Autodesk Inventor part; units mm, degrees
ref_plane "YZ Plane" through (0, 0, 0) normal (1, 0, 0) x (0, 1, 0)
ref_plane "XZ Plane" through (0, 0, 0) normal (0, 1, 0) x (-1, 0, 0)
ref_plane "XY Plane" through (0, 0, 0) normal (0, 0, 1) x (1, 0, 0)
sketch "Sketch1" plane through (0, 0, 0) normal (0, 0, 1) x (1, 0, 0)
  line L0 (-20, 10) -> (20, 10)
  line L1 (20, 10) -> (20, -10)
  line L2 (20, -10) -> (-20, -10)
  line L3 (-20, -10) -> (-20, 10)
  line L4 (-20, 10) -> (20, -10) construction
  line L5 (20, 10) -> (-20, -10) construction
  line L6 (18, 8) -> (-18, 8)
  line L7 (-18, 8) -> (-18, -8)
  line L8 (-18, -8) -> (18, -8)
  line L9 (18, -8) -> (18, 8)
  point P0 (0, 0)
  dimension "d0" = 40
  dimension "d1" = 20
  dimension "d2" = 2
extrude "Extrusion1" add sketch "Sketch1" along normal mid plane 1900
sketch "Sketch2" plane through (0, 0, 0) normal (0, 1, 0) x (-1, 0, 0)
  line L0 (20, -950) -> (20, 950)
  line L1 (-20, 950) -> (20, 950)
  line L2 (-20, -950) -> (-20, 950)
  line L3 (20, -950) -> (-20, -950)
  line L4 (-20, -950) -> (-50.7107, -950)
  line L5 (-50.7107, -950) -> (-50.7107, 950)
  line L6 (-50.7107, 950) -> (-20, 950)
  line L7 (20, -879.2893) -> (-50.7107, -950)
  line L8 (20, -879.2893) -> (-20, -862.7208)
  line L9 (-20, -950) -> (-20, 950)
  point P0 (0, 0)
  point P1 (-20, -919.2893)
  dimension "d5" = 45
  dimension "d6" = 100
  dimension "d19" = 67.5
extrude "Extrusion2" cut sketch "Sketch2" along normal through all both and the other way through all contours L3 L2 L7 L0 | L7 L2 L8
mirror "Mirror1" about plane through (0, 0, 0) normal (0, 0, 1) of "Extrusion2"
sketch "Sketch3" plane through (0, 0, 0) normal (0, 1, 0) x (-1, 0, 0)
  line L0 (0, 0) -> (0, -871.0051) construction
  line L1 (-20, -862.7208) -> (-20, 862.7208) construction
  line L2 (-20, -475) -> (20, -475) construction
  line L3 (20, 879.2893) -> (20, -879.2893) construction
  circle A0 centre (0, -100) radius 5.5
  circle A1 centre (0, -375) radius 5.5
  circle A2 centre (0, -575) radius 5.5
  circle A3 centre (0, -850) radius 5.5
  line L4 (20, 879.2893) -> (20, -879.2893) construction
  line L5 (-20, -862.7208) -> (20, -879.2893) construction
  dimension "d9" = 475
  dimension "d10" = 11
  dimension "d11" = 275
  dimension "d12" = 275
  dimension "d13" = 100
  dimension "d14" = 100
  dimension "d15" = 100
extrude "Extrusion3" cut sketch "Sketch3" along normal through all
sketch "Sketch5" plane through (-20, -10, -879.2893) normal (0, -1, 0) x (1, 0, 0)
  line L0 (40, 1742.0101) -> (0, 1758.5786) construction
  line L1 (0, 1758.5786) -> (0, 0) construction
  line L2 (0, 0) -> (40, 16.5685) construction
  line L3 (40, 16.5685) -> (40, 1742.0101) construction
  circle A0 centre (20, 114.2893) radius 5.5
  circle A1 centre (20, 760.7893) radius 5.5
  circle A2 centre (20, 285.7893) radius 5.5
  circle A3 centre (20, 522.7893) radius 5.5
  line L4 (20, 522.7893) -> (20, 285.7893) construction
  point P0 (20, 879.2893)
  point P1 (20, 8.2843)
  point P2 (20, 404.2893)
  dimension "d20" = 765
  dimension "d21" = 11
  dimension "d24" = 11
  dimension "d25" = 118.5
  dimension "d26" = 237
  dimension "d27" = 475
extrude "Extrusion4" cut sketch "Sketch5" against normal up to surface (2 mm away)
mirror "Mirror2" about plane through (0, 0, 0) normal (0, 0, 1) of "Extrusion3", "Extrusion4"
fillet "Fillet1" radius 2 4 edges at (-20, 10, 0) (-20, -10, 0) (20, -10, 0) (20, 10, 0)
equation "\"d19\" = 1.5 * d5"
equation "\"d11\" = d12"
equation "\"d13\" = d15"
equation "\"d14\" = d15"
properties part number "Long tube 1"
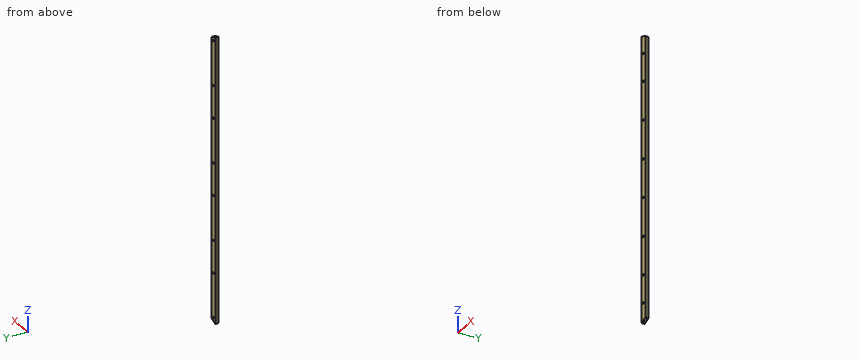
Verification items for the finished model (mm, model axes). Round coordinates to 2 decimals unless told otherwise and drop trailing zeros. Order: outer loops, then holes, each group sorted by start corner. A loop starts at its lowest first (then second) coordinate and runs counter-clockwise, first axis right, second up. Notation, with made-up numbers: (25.5, -21) - (83.5, -21) arc R33 ccw to (83.5, 9) - close; hole circle Ø9 at (21, -25.5). An arc over 180 degrees is marked (long way). Use CSV: the item, a comma, the result in double quotes. Start each with the question number.
1) Go/stop test with flat-tipped pins: P1, Ø10, axis at x = 0, z = -118.5, coming from the -Y side; P2, Ø9, axis at x = 0, z = 100, coming from the +Y side. Record where each tip stops, or that it passes through.
2) Thickness scan on L1, parallel to X at y = -7.75, z = -23; L2, parallel to Y at x = 17, z = 270.5; L3, parallel to X at y = 8.7, z = -850. Record the ranges inside material, lowest first.
3) Section check B-B, the plane z = -688.5. Record the cut outline in (x, y), plus the area to 3 significant figures.
4) Section check A-A, the plane y = -3.5. Record the cut outline in (x, z), plus the area to 3 significant figures.
Answers:
1,P1,"stops at y = 8"
1,P2,"stops at y = -8"
2,L1,"x = -20 to -18, 18 to 20"
2,L2,"y = -10 to -8, 8 to 10"
2,L3,"x = -19.87 to -5.5, 5.5 to 19.87"
3,outline,"(-20, -8) arc R2 ccw to (-18, -10) - (18, -10) arc R2 ccw to (20, -8) - (20, 8) arc R2 ccw to (18, 10) - (-18, 10) arc R2 ccw to (-20, 8) - close; hole (-18, -8) - (18, -8) - (18, 8) - (-18, 8) - close"
3,area,"221 mm²"
4,outline,"(-20, -879.29) - (-18, -878.46) - (-18, 878.46) - (-20, 879.29) - close; (18, -863.55) - (20, -862.72) - (20, 862.72) - (18, 863.55) - close"
4,area,"6,970 mm²"
